Can you work these out from the drawing? Everything is in mm from the part's minimum corner. Coordinates: 2 decimals unless noted, no trailing zeros. Order: outer loops, then holes, each group sorted by start corner. A loop starts at its lowest first (then second) coordinate and runs counter-clockwise, first axis right, second up. Notation, with made-up numbers: (85.25, -1) - (120.25, -1) arc R14 cw to (120.25, 26) - close; hole circle Ø9 at (63.25, 81). An arc over 180 degrees is marked (long way). Use a Markdown table: item, result. Add a question column.
(1) I want a section at C-C (x = 25). List the corners of the cut face in (y, z) for me.
(2) I want a section at D-D (x = 15.5). List the corners of the cut face in (y, z) for me.
(3) I want a section at A-A (y = 2.7). List the corners of the cut face in (x, z) for me, and give its area (3 significant figures).
(4) We'd pull the mould along X, two halves only. Please class the marked faces 1, 2 and 3: pulls with the +X half, pulls with the -X half, needs draft (parallel to the pull), parting line crosses it, or undercut.
(5) If I drill on L1, parallel to X at y = 0.75, z = 5.5; L2, parallel to X at y = 2.9, z = 40; L3, parallel to Y at x = 25, z = 25.5, over which ranges is the centre line in solid material (lowest first)? Write a range as [from, to].
(6) I want a section at B-B (z = 21). List the corners of the cut face in (x, y) for me, and give its area (3 significant figures).
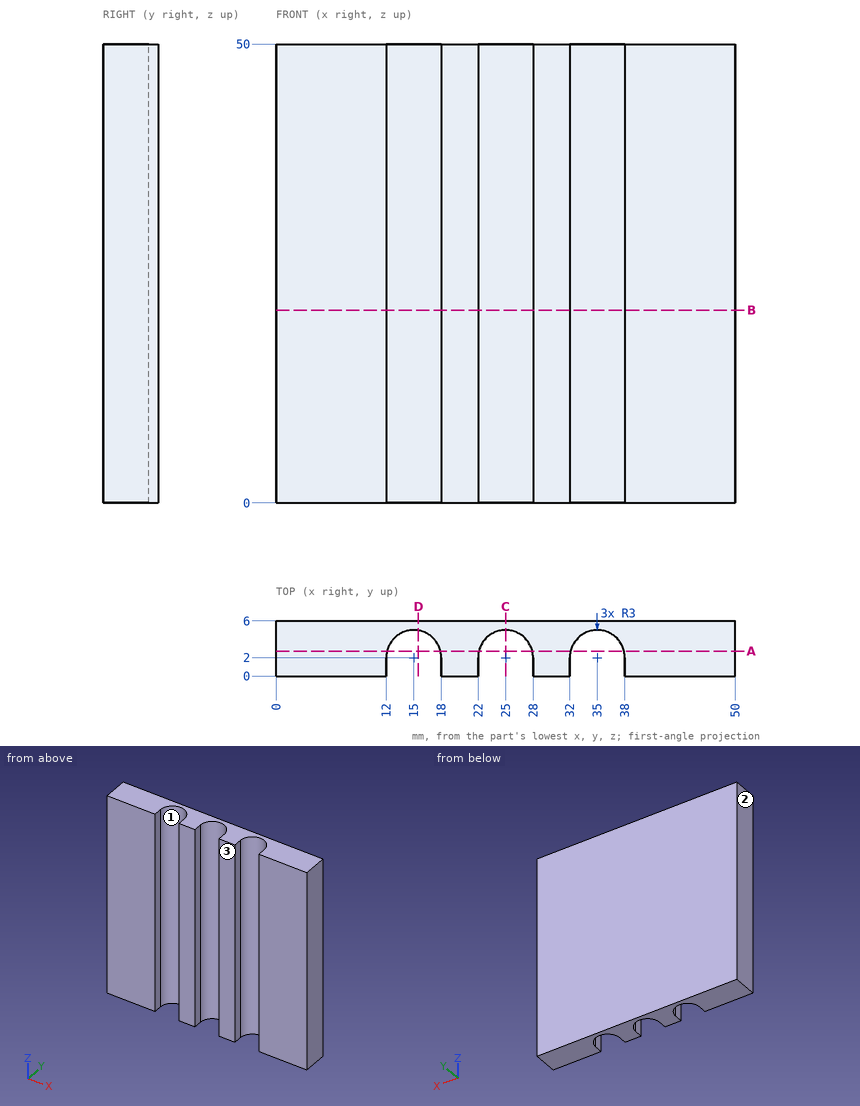
Answers follow:
| question | item | result |
|---|---|---|
| 1 | outline | (5, 0) - (6, 0) - (6, 50) - (5, 50) - close |
| 2 | outline | (4.96, 0) - (6, 0) - (6, 50) - (4.96, 50) - close |
| 3 | outline | (0, 0) - (12.08, 0) - (12.08, 50) - (0, 50) - close; (17.92, 0) - (22.08, 0) - (22.08, 50) - (17.92, 50) - close; (27.92, 0) - (32.08, 0) - (32.08, 50) - (27.92, 50) - close; (37.92, 0) - (50, 0) - (50, 50) - (37.92, 50) - close |
| 3 | area | 1,620 mm² |
| 4 | face 1 | undercut |
| 4 | face 2 | pulls with the -X half |
| 4 | face 3 | needs draft |
| 5 | L1 | x = [0, 12], [18, 22], [28, 32], [38, 50] |
| 5 | L2 | x = [0, 12.14], [17.86, 22.14], [27.86, 32.14], [37.86, 50] |
| 5 | L3 | y = [5, 6] |
| 6 | outline | (0, 0) - (12, 0) - (12, 2) arc R3 cw to (18, 2) - (18, 0) - (22, 0) - (22, 2) arc R3 cw to (28, 2) - (28, 0) - (32, 0) - (32, 2) arc R3 cw to (38, 2) - (38, 0) - (50, 0) - (50, 6) - (0, 6) - close |
| 6 | area | 222 mm² |
